```python
from build123d import *

# Parameters (mm, degrees)
BOSS_EXTRUDE1_DEPTH = 25.4
SHELL1_T            = -1.5875
SKETCH2_R           = 1.771315789
CUT_EXTRUDE1_DEPTH  = 224.468749705


with BuildPart() as part:
    # Sketch1 → Boss-Extrude1 (new body)
    with BuildSketch(Plane.XY):
        Polygon((171.8384328, 137.597905652), (-22.225, 39.800277228), (-22.225, 28.575), (3.175, 28.575), (3.175, 3.175), (17.979241427, 3.175), (174.241035508, 81.922616972), align=None)
    extrude(amount=BOSS_EXTRUDE1_DEPTH)

    # Shell1
    shell1_openings = [part.faces().sort_by_distance(p)[0] for p in [
        (10.577120713, 3.175, 12.7),
        (3.175, 15.875, 12.7),
        (-9.525, 28.575, 12.7),
        (-22.225, 34.187638614, 12.7),
        (173.039734154, 109.760261312, 12.7),
    ]]
    offset(amount=SHELL1_T, openings=shell1_openings, kind=Kind.INTERSECTION)

    # Sketch2 → Cut-Extrude1 (cut, through all)
    with BuildSketch(Plane.XY.offset(25.4)):
        with Locations((2.461305961, 27.861305961)):
            Circle(SKETCH2_R)
    extrude(amount=-CUT_EXTRUDE1_DEPTH, mode=Mode.SUBTRACT)


solid = part.part
```
Here's how the part is built. I have some questions about the finished solid (model axes, mm). A direction names the side the tool comes from. Give positions to 0.01 mm unless a question says otherwise; leave off trailing zeros. Write each loop counter-clockwise with the first axis right and the second up, starting at its lowest first coordinate (ties: lowest second). Pieces come first, ordered by that corner, then holes. Notation, with made-up numbers: M 33,57 L 88,57 A21 ccw 88,92 Z; hole C -31.75,-18 d4. An arc over 180 degrees is marked long. Put each result on its own line as item: value. Start each with the question number.
Item 1: I need wall thicknesses on L1, parallel to Z at x = 30, y = 61; L2, parallel to Y at x = 108, z = 14.5; L3, parallel to Y at x = 45, z = 12. Which ranges of each line are inside material? Lowest first, please. Write a range as from..to.
Item 2: Thinking about a two-plate mould opening in Z: for faces 3 (the flat face through (76.2, 89.4, 12.5)), 4 (the flat face through (75, 71, 0)), 5 (the flat face through (93.191, 42.855, 12.544)), which applies, +Z half, -Z half, draft (parallel to the pull), parting line (faces both ways), or undercut?
Item 3: Will these pins go through, and if not, where does the flat tip stop? pin 1 (2 mm diameter, centred on x = 144.5, z = 14, fed in from +Y); pin 2 (1.7 mm diameter, centred on y = 19.5, z = 1, fed in from -X) (3 decimals); pin 3 (6 mm diameter, centred on x = 69, z = 17.5, fed in from -Y).
Item 4: If we section it at A-A, the plane z = 6.25: Write out the boundary of the cut face in (x, y) (3 decimals).
Item 5: If we section it at C-C, the plane x = 159.5: Write out the boundary of the cut face in (y, z).
Item 6: If we section it at D-D, the plane x = -10: Write out the boundary of the cut face in (y, z) (1 decimal), then the cut area to 3 significant figures.
Item 7: On a 3-axis mill with a long thin cutter (end or side, diameter ignored), from which of +Z, -Z, +X, -X, +Y, -Y can I reach the whole of each face in a straight line? I mean faces 1 (the flat face through (76.203, 87.625, 12.544)), 2 (the flat face through (15, 3.175, 14)). Say none if no direction works.
Item 8: If we section it at B-B, the plane y = 128: Write out the boundary of the cut face in (x, z).
Values:
1. L1: 0..1.59, 23.81..25.4
1. L2: 48.54..50.32, 103.65..105.43
1. L3: 16.79..18.57, 71.9..73.68
2. face 3: draft
2. face 4: -Z half
2. face 5: undercut
3. pin 1: y = 124.32
3. pin 2: x = 3.175
3. pin 3: y = 27.37
4. outline: M -22.225,38.023 L 171.914,135.858 L 171.838,137.598 L -22.225,39.8 Z; M 14.452,3.175 L 17.979,3.175 L 174.241,81.923 L 174.166,83.662 Z
5. outline: M 74.49,0 L 131.38,0 L 131.38,25.4 L 74.49,25.4 Z; hole M 76.27,1.59 L 129.6,1.59 L 129.6,23.81 L 76.27,23.81 Z
6. outline: M 28.6,0 L 46,0 L 46,25.4 L 28.6,25.4 L 28.6,23.8 L 44.2,23.8 L 44.2,1.6 L 28.6,1.6 Z
6. area: 94.7 mm²
7. face 1: none
7. face 2: +Z, -Z, +X, -X, -Y
8. outline: M 152.79,0 L 172.25,0 L 172.25,1.59 L 156.32,1.59 L 156.32,23.81 L 172.25,23.81 L 172.25,25.4 L 152.79,25.4 Z
